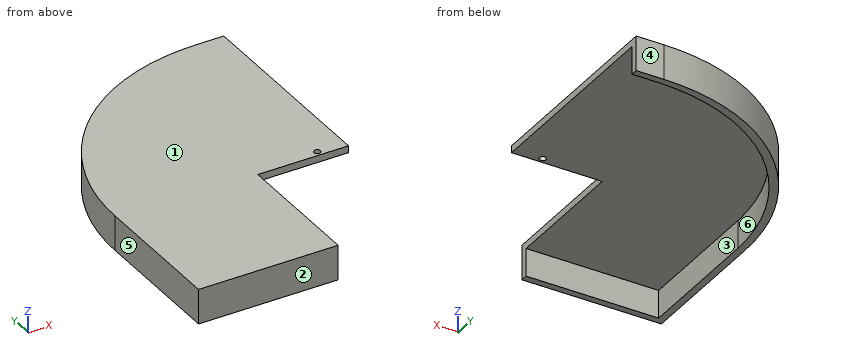
Autodesk Inventor part; units mm, degrees
ref_plane "YZ Plane" through (0, 0, 0) normal (1, 0, 0) x (0, 1, 0)
ref_plane "XZ Plane" through (0, 0, 0) normal (0, 1, 0) x (-1, 0, 0)
ref_plane "XY Plane" through (0, 0, 0) normal (0, 0, 1) x (1, 0, 0)
ref_plane "Work Plane1" through (0, 0, 0) normal (0, 0, 1) x (1, 0, 0)
sketch "Sketch1" plane through (0, 0, 0) normal (0, 0, 1) x (1, 0, 0)
  circle A0 centre (0, -114.3) radius 4 construction
  line L0 (0, -114.3) -> (-57.15, -114.3) construction
  line L1 (0, -114.3) -> (0, 63.5) construction
  line L2 (25.4, 69.85) -> (0, 69.85)
  arc A1 (0, 69.85) -> (-184.15, -114.3) centre (0, -114.3) ccw
  line L3 (25.4, 69.85) -> (25.4, -114.3)
  line L4 (-184.15, -114.3) -> (-184.15, -241.3)
  line L5 (-184.15, -241.3) -> (-57.15, -241.3)
  line L6 (-57.15, -241.3) -> (-57.15, -119.38)
  line L7 (-57.15, -114.3) -> (-177.8, -114.3) construction
  line L8 (25.4, -114.3) -> (25.4, -119.38)
  line L9 (25.4, -119.38) -> (-57.15, -119.38)
  circle A2 centre (0, -114.3) radius 4
  point P0 (0, 0)
  dimension "d1" = 90
  dimension "d4" = 25.4
  dimension "d5" = 184.15
  dimension "d6" = 127
  dimension "d7" = 127
  dimension "d16" = 5.08
extrude "Extrusion1" add sketch "Sketch1" along normal blind 6.35 contours L3 L8 L9 L6 L5 L4 A1 L2 | A2
sketch "Sketch2" plane through (0, 0, 0) normal (0, 0, -1) x (-1, 0, 0)
  arc A0 (184.15, -114.3) -> (0, 69.85) centre (0, -114.3) ccw
  line L0 (-25.4, 69.85) -> (0, 69.85) construction
  arc A1 (184.15, -114.3) -> (0, 69.85) centre (0, -114.3) ccw construction
  line L1 (-25.4, -119.38) -> (-25.4, 69.85) construction
  line L2 (0, 69.85) -> (-25.4, 69.85) construction
  line L3 (-25.4, 69.85) -> (-25.4, 63.5) construction
  line L4 (-25.4, 63.5) -> (0, 63.5)
  line L5 (0, 63.5) -> (-25.4, 63.5) construction
  line L6 (-25.4, 69.85) -> (0, 69.85)
  line L7 (-25.4, 63.5) -> (-25.4, 69.85)
  line L8 (-25.4, 69.85) -> (0, 69.85)
  arc A2 (177.8, -114.3) -> (0, 63.5) centre (-3.1476, -117.4476) ccw
  line L9 (184.15, -114.3) -> (184.15, -241.3)
  line L10 (184.15, -114.3) -> (184.15, -241.3)
  line L11 (184.15, -241.3) -> (57.15, -241.3)
  line L12 (184.15, -241.3) -> (57.15, -241.3)
  line L13 (57.15, -241.3) -> (57.15, -234.95)
  line L14 (57.15, -241.3) -> (57.15, -119.38)
  line L15 (57.15, -234.95) -> (177.8, -234.95)
  line L16 (177.8, -234.95) -> (177.8, -114.3)
  point P0 (0, 0)
  point P1 (-25.4, -114.3)
  point P2 (57.15, -114.3)
  dimension "d10" = 6.35
  dimension "d11" = 6.35
  dimension "d12" = 180.975
  dimension "d13" = 6.35
extrude "Extrusion2" add sketch "Sketch2" along normal blind 25.4
sketch "Sketch3" plane through (0, 0, 6.35) normal (0, 0, 1) x (1, 0, 0)
  arc A0 (-2.982, -113.9716) -> (-0.8571, -111.4251) centre (0, -114.3) ccw construction
  circle A1 centre (0, -114.3) radius 3
  point P0 (0, 0)
extrude "Extrusion3" cut sketch "Sketch3" against normal through all
properties part number "Ring Shooter guide"
For this review, take the finished solid that the model builds, in its own axes (mm). Face numbers are marked on the shaded views. A direction names the side the tool comes from. Coordinates: 2 decimals unless noted, no trailing zeros. Write each loop counter-clockwise with the first axis right and the second up, starting at its lowest first coordinate (ties: lowest second). Pieces come first, ordered by that corner, then holes. Notation, with made-up numbers: (26.5, -27) - (61.5, -27) arc R15 ccw to (61.5, -4) - close; hole circle Ø10 at (68.25, -39). An arc over 180 degrees is marked (long way). Answer in a Markdown table with one row per item. Add a question column.
Q1. We need section B-B, the plane y = -135.5. State the section outline as (x, z) points, and give its area (3 significant figures).
Q2. For P1, Ø3, axis at x = -43.5, z = -19.5, coming from the +Y side; P2, Ø1.5, axis at y = -80, z = -10.5, coming from the +X side; P3, Ø5, axis at x = -8.5, z = 3.5, coming from the -Y side; P4, Ø5.5, axis at x = 0, y = -114.3, coming from the -Z side, all flat-tipped, find the tip position at first contact; note any pin that passes through.
Q3. We need section D-D, the plane x = -68. State the section outline as (y, z) points.
Q4. We need section A-A, the plane z = -8. State the section outline as (x, y) points.
Q5. For probe 1 along Y at (x, z) = (0, 4); probe 2 along Z at (x, y) = (-40.5, -74.5); probe 3 along X at (y, z) = (-114, 2), list the stretches that pass through material, from the lowest coordinate up.
Q6. We need section C-C, the plane x = -110. State the section outline as (y, z) points.
Q7. Draft analysis for pull direction Y (two halves, no side actions). For the marked faces 1, 2, 3 and 4, state which applies: +Y half, -Y half, draft (parallel to the pull), parting line (faces both ways), or undercut.
Q8. Tool access review of the marked faces 5 and 6: name each direction out of +Z, -Z, +X, -X, +Y, -Y from which nothing blocks a thin tool from reaching the whole face with its end or side.
Answer list:
| question | item | result |
|---|---|---|
| 1 | outline | (-184.15, -25.4) - (-177.8, -25.4) - (-177.8, 0) - (-57.15, 0) - (-57.15, 6.35) - (-184.15, 6.35) - close |
| 1 | area | 968 mm2 |
| 2 | P1 | stops at y = 65 |
| 2 | P2 | stops at x = -173.75 |
| 2 | P3 | stops at y = -119.38 |
| 2 | P4 | passes through |
| 3 | outline | (-241.3, -25.4) - (-234.95, -25.4) - (-234.95, 0) - (48.96, 0) - (48.96, -25.4) - (56.84, -25.4) - (56.84, 6.35) - (-241.3, 6.35) - close |
| 4 | outline | (-184.15, -241.3) - (-57.15, -241.3) - (-57.15, -234.95) - (-177.8, -234.95) - (-177.8, -114.3) arc R180.97 cw to (0, 63.5) - (25.4, 63.5) - (25.4, 69.85) - (0, 69.85) arc R184.15 ccw to (-184.15, -114.3) - close |
| 5 | probe 1 | y = -119.38 to -117.3, -111.3 to 69.85 |
| 5 | probe 2 | z = 0 to 6.35 |
| 5 | probe 3 | x = -184.15 to -2.98, 2.98 to 25.4 |
| 6 | outline | (-241.3, -25.4) - (-234.95, -25.4) - (-234.95, 0) - (23.8, 0) - (23.8, -25.4) - (33.39, -25.4) - (33.39, 6.35) - (-241.3, 6.35) - close |
| 7 | face 1 | draft |
| 7 | face 2 | -Y half |
| 7 | face 3 | undercut |
| 7 | face 4 | +Y half |
| 8 | face 5 | +Z, -Z, -X, +Y, -Y |
| 8 | face 6 | -Z, +X |
